Could you check a few things on this model? Use its own coordinates, in mm. Face numbers are marked on the shaded views. A direction names the side the tool comes from. Round coordinates to 2 decimals unless told otherwise and drop trailing zeros. Write each loop counter-clockwise with the first axis right and the second up, starting at its lowest first coordinate (ties: lowest second). Pieces come first, ordered by that corner, then holes. Notation, with made-up numbers: (-37, 39.5) -> (12, 39.5) arc R27 ccw to (12, 60.5) -> close; hole circle Ø8 at (26, 42.25). An arc over 180 degrees is marked (long way). Answer in a Markdown table with one row per item. Add a question column.
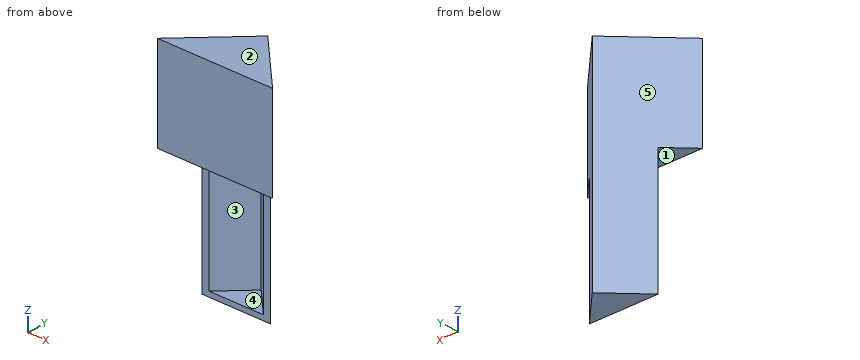
```python
from build123d import *

# Parameters (mm, degrees)
F1_DEPTH = 1219.2
F3_DEPTH = 914.4
F4_T     = 50.8


# Not quite as in the source:
# - a shell that OpenCascade refuses in one call is made with other operations: the cavity is built on its own and cut out


with BuildPart() as f1:
    # F0 (on Top) → F1 (new body)
    with BuildSketch(Plane.XY):
        Polygon((0, 0), (-341.2497326006, -341.2497326006), (341.2497326006, -341.2497326006), align=None)
    extrude(amount=F1_DEPTH)

    # F2 (on face) → F3 (join)
    with BuildSketch(Plane.XY.offset(1219.2)):
        Polygon((341.2497326006, -341.2497326006), (0, 0), (-341.2497326006, -341.2497326006), align=None)
        Polygon((341.2497326006, -341.2497326006), (-341.2497326006, -341.2497326006), (-571.5, -571.5), (571.5, -571.5), align=None)
    extrude(amount=F3_DEPTH)

    # F4: shell of thickness 50.8, made by hand


with BuildPart() as f4_core1:
    # F4_t2: copy of F1
    add(f1.part)

    # the walls: a layer under each face that stays
    f4_faces = [f4_core1.faces().sort_by_distance(p)[0] for p in [
        (-285.75, -285.75, 1066.8),
        (0, -170.6248663003, 0),
        (0, -456.3748663003, 1219.2),
        (0, -571.5, 1676.4),
        (0, -285.75, 2133.6),
        (285.75, -285.75, 1066.8),
    ]]
    thicken(f4_faces, amount=-F4_T, mode=Mode.SUBTRACT)


with BuildPart() as f1_1:
    add(f1.part)

    # what is left inside the walls is the cavity
    f4_cavity = [f4_core1.part.solids().sort_by_distance(p)[0] for p in [
        (-224.069765, -296.630235, 1405.466667),
    ]]
    add(f4_cavity, mode=Mode.SUBTRACT)


solid = f1_1.part
```
(1) Suppose I cut it at C-C, the plane x = 407. Please give me the cut outline in (y, z).
(2) I need wall thicknesses on L1, parallel to Z at x = -58, y = -505; L2, parallel to Z at x = -89, y = -184.5; L3, parallel to Y at x = -162, z = 1519. Which ranges of each line are inside material? Lowest first, please.
(3) For P1, Ø10, axis at x = -196.5, z = 1405, coming from the +Y side; P2, Ø8, axis at x = 73.5, z = 837.5, coming from the +Y side; P3, Ø1, axis at y = -179, z = 914, coming from the -X side, each with a flat end and sliding along its axis, tell me the tip position at first contact or that it passes through.
(4) Suppose I cut it at A-A, the plane y = -407.5. Please give me the cut outline in (x, z).
(5) Suppose I cut it at D-D, the plane z = 1197. Please give me the cut outline in (x, y), then the cut area to 3 significant figures.
(6) If we mould it in two halves opening along Y, with no side actions, what happens to the marked faces 3, 4 and 5? For each: pulls with the +Y half, pulls with the -Y half, needs draft (parallel to the pull), parting line crosses it, or undercut.
(7) On a 3-axis mill with a long thin cutter (end or side, diameter ignored), from which of +Z, -Z, +X, -X, +Y, -Y can I reach the whole of each face in a straight line? I mean the marked faces 1 and 2. Say none if no direction works.
(8) Suppose I cut it at B-B, the plane z = 1665. Please give me the cut outline in (x, y), then the cut area to 3 significant figures.
Response:
| question | item | result |
|---|---|---|
| 1 | outline | (-571.5, 1219.2) -> (-407, 1219.2) -> (-407, 2133.6) -> (-571.5, 2133.6) -> close; hole (-520.7, 1270) -> (-478.84, 1270) -> (-478.84, 2082.8) -> (-520.7, 2082.8) -> close |
| 2 | L1 | 1219.2 to 1270, 2082.8 to 2133.6 |
| 2 | L2 | 0 to 50.8, 2082.8 to 2133.6 |
| 2 | L3 | -571.5 to -520.7, -233.84 to -162 |
| 3 | P1 | y = -191.5 |
| 3 | P2 | y = -69.5 |
| 3 | P3 | x = -179.5 |
| 4 | outline | (-407.5, 1219.2) -> (407.5, 1219.2) -> (407.5, 2133.6) -> (-407.5, 2133.6) -> close; hole (-335.66, 1270) -> (335.66, 1270) -> (335.66, 2082.8) -> (-335.66, 2082.8) -> close |
| 5 | outline | (-341.25, -341.25) -> (-269.41, -341.25) -> (0, -71.84) -> (269.41, -341.25) -> (341.25, -341.25) -> (0, 0) -> close |
| 5 | area | 43,900 mm² |
| 6 | face 3 | undercut |
| 6 | face 4 | needs draft |
| 6 | face 5 | pulls with the +Y half |
| 7 | face 1 | -Z, +X, -X, -Y |
| 7 | face 2 | +Z, +X, -X, +Y, -Y |
| 8 | outline | (-571.5, -571.5) -> (571.5, -571.5) -> (0, 0) -> close; hole (-448.86, -520.7) -> (448.86, -520.7) -> (0, -71.84) -> close |
| 8 | area | 125,000 mm² |
